For this review, use the dimensioned drawing (mm, ordinates from the lowest corner) and the shaded views. A direction names the side the tool comes from. Round coordinates to 2 decimals unless told otherwise and drop trailing zeros. Order: outer loops, then holes, each group sorted by start corner. A loop starts at its lowest first (then second) coordinate and runs counter-clockwise, first axis right, second up. Notation, with made-up numbers: (69.5, 41) - (114.5, 41) arc R11 cw to (114.5, 45) - close; hole circle Ø11 at (-21.75, 20.25). An arc over 180 degrees is marked (long way). Write each question's results on one line, items separated by ' | '. Start each with the question number.
(1) Take a section at C-C, the plane x = 40. Give the boundary of the cut face in (y, z), plus the area to 3 significant figures.
(2) Take a section at B-B, the plane z = 99. Give the boundary of the cut face in (x, y) (1 decimal).
(3) Draft analysis for pull direction Z (two halves, no side actions). For the marked faces 3, 4 and 5, state which applies: pulls with the +Z half, pulls with the -Z half, needs draft (parallel to the pull), parting line crosses it, or undercut.
(4) For the marked faces 1 and 2, list the 3-axis set-ups (+Z, -Z, +X, -X, +Y, -Y) from which the entire face can be reached by the end or side of a thin tool; tool diameter is ignored.
(5) Take a section at D-D, the plane y = 15. Give the boundary of the cut face in (x, z) (1 decimal), plus the area to 3 significant figures.
(6) Take a section at A-A, the plane y = 41.5. Give the boundary of the cut face in (x, z) (1 decimal), plus the area to 3 significant figures.
(7) For L1, parallel to X at y = 36.5, z = 31 (1 decimal); L2, parallel to Y at x = 93.5, z = 48.5; L3, parallel to X at y = 32.5, z = 81 (1 decimal), list the stretches that pass through material, from the lowest coordinate up. Write a range as from..to.
(8) Insertion check: pin 1 Ø8 at (y, z) = (27, 69) entering from +X (1 decimal); pin 2 Ø6 at (x, z) = (136.5, 89.5) entering from -Y; pin 3 Ø5 at (y, z) = (28.5, 39) entering from +X (1 decimal); pin 4 Ø12 at (x, y) = (53.5, 22.5) entering from +Z. Each pin has a flat end and moves straight along its axis. Give the tip position at first contact, or say it passes through.
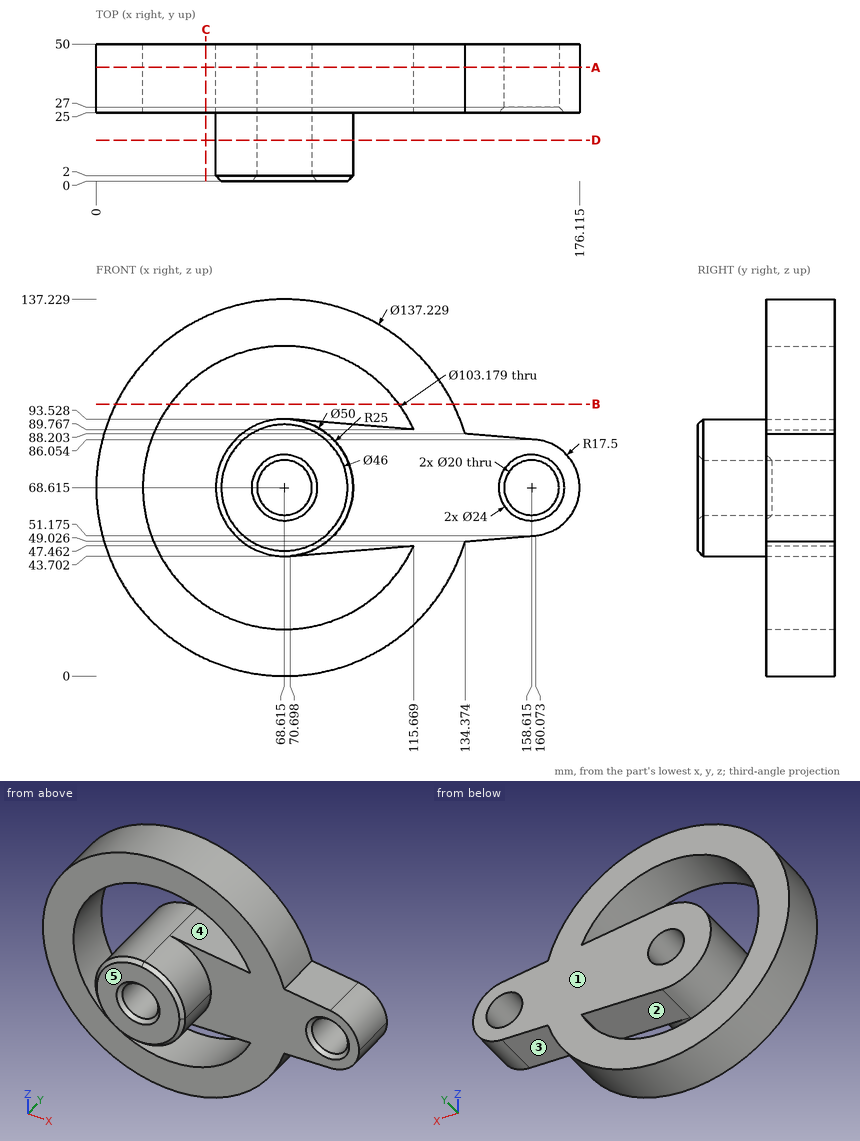
Results below:
1) outline: (25, 6.25) - (50, 6.25) - (50, 25.69) - (25, 25.69) - close; (25, 111.54) - (50, 111.54) - (50, 130.98) - (25, 130.98) - close | area: 972 mm^2
2) outline: (7.1, 25) - (26.9, 25) - (26.9, 50) - (7.1, 50) - close; (110.3, 25) - (130.1, 25) - (130.1, 50) - (110.3, 50) - close
3) face 3: pulls with the -Z half | face 4: undercut | face 5: needs draft
4) face 1: +Z, -Z, +X, -X, +Y | face 2: +Y, -Y
5) outline: (70.7, 43.7) arc R25 ccw to (93.6, 68.6) arc R25 ccw to (70.7, 93.5) arc R25 ccw (long way) to start; hole circle Ø20 at (68.6, 68.6) | area: 1,650 mm^2
6) outline: (134.4, 49) - (160.1, 51.2) arc R17.5 ccw to (160.1, 86.1) - (134.4, 88.2) arc R68.6 ccw (long way) to start; hole circle Ø20 at (68.6, 68.6); hole (70.7, 43.7) arc R25 cw (long way) to (70.7, 93.5) - (115.7, 89.8) arc R51.6 ccw (long way) to (115.7, 47.5) - close; hole circle Ø20 at (158.6, 68.6) | area: 10,400 mm^2
7) L1: x = 11.2..33.3, 103.9..126 | L2: y = 25..50 | L3: x = 1.1..18.5, 46.9..171
8) pin 1: stops at x = 176.1 | pin 2: stops at y = 25 | pin 3: stops at x = 131.6 | pin 4: stops at z = 136.55
